Source: CAD feature listing. Evaluate the final solid. Frame: model axes, mm. A direction names the side the tool comes from. Round coordinates to 2 decimals unless told otherwise and drop trailing zeros. Write each loop counter-clockwise with the first axis right and the second up, starting at its lowest first coordinate (ties: lowest second). Pieces come first, ordered by that corner, then holes. Notation, with made-up numbers: M 36.5,-33.75 L 54.5,-33.75 A29 ccw 54.5,-9.75 Z; hole C 15.5,69 d10. An arc over 180 degrees is marked long. Answer in a Markdown table with one row per item. Add a question column.
Item 1: Cut plane A-A on y = -27. Return loops of the section in (x, z).
Item 2: Cut plane C-C on x = 4. Return loops of the section in (y, z).
Item 3: Mould query, pull axis Z, two halves, no side actions, for faces 4 (the face through (24, 20, 19)), 5 (the face through (25, 0, 37)), 6 (the face through (6.141, -0.224, 38.797)). Classes: released by +Z, released by -Z, zero draft, split by the parting line, or undercut.
Item 4: Cut plane B-B on x = 35. Give the number of separate pieces and of enclosed holes in the cut face, and give its area (3 significant figures).
Item 5: Material intervals for probe 1 along Y at (x, z) = (4, 9.25); probe 2 along Y at (x, z) = (21.5, 21.5); probe 3 along Z at (x, y) = (7, -21), sorted ascending.
Item 6: Cut plane D-D on y = 10. Return loops of the section in (x, z).
Item 7: Set-up query: faces 1 (the face through (31, 5, 41)), 2 (the face through (39, -5, 41)), 3 (the face through (8, -27, 9)). Return all of +Z, -Z, +X, -X, +Y, -Y with unobstructed straight access to the full face (end or side cutting, diameter ignored); none if empty.
Item 8: Contact query for flat-ended pins moving along their axis: pin 1 (5 mm diameter, centred on x = 7, y = 1, fed in from +Z); pin 2 (1.5 mm diameter, centred on y = 18, z = 19, fed in from -X); pin 3 (2 mm diameter, centred on y = 3.5, z = 41.5, fed in from -X). Output: stop coordinate, or through.
from build123d import *

# Parameters (mm, degrees)
ESTRUSIONE_ESTRUSIONE1_DEPTH  = 10
SCHIZZO6_W                    = 8
SCHIZZO6_H                    = 8
SCHIZZO6_H_2                  = 2
ESTRUSIONE_ESTRUSIONE4_DEPTH  = 10
TAGLIO_ESTRUSIONE1_DEPTH      = 54.150729064
SCHIZZO4_W                    = 3
SCHIZZO4_H                    = 6
ESTRUSIONE_ESTRUSIONE2_DEPTH  = 3
SCHIZZO5_W                    = 3
SCHIZZO5_H                    = 6
ESTRUSIONE_ESTRUSIONE3_DEPTH  = 3
SCHIZZO3_W                    = 5
SCHIZZO3_H                    = 6
TAGLIO_ESTRUSIONE2_DEPTH      = 67.820655489
FORO_FILETTATO_M3X0_5_1_D     = 2.5
ESTRUSIONE_ESTRUSIONE5_DEPTH  = 30
SCHIZZO10_W                   = 3
SCHIZZO10_H                   = 34
ESTRUSIONE_ESTRUSIONE6_DEPTH  = 34
SCHIZZO18_W                   = 8
SCHIZZO18_H                   = 8
TAGLIO_ESTRUSIONE3_DEPTH      = 5
SCHIZZO24_W                   = 8
SCHIZZO24_H                   = 2
ESTRUSIONE_ESTRUSIONE9_DEPTH  = 5
SCHIZZO23_W                   = 8
SCHIZZO23_H                   = 8
TAGLIO_ESTRUSIONE4_DEPTH      = 5
SCHIZZO25_W                   = 8
SCHIZZO25_H                   = 2
ESTRUSIONE_ESTRUSIONE10_DEPTH = 5
FORO_FILETTATO_M3X0_5_4_D     = 2.5
FORO_FILETTATO_M3X0_5_4_DEPTH = 7.5
FORO_FILETTATO_M3X0_5_4_TIP   = 0.751075774
FORO_FILETTATO_M3X0_5_5_D     = 2.5
FORO_FILETTATO_M3X0_5_5_DEPTH = 7.5
FORO_FILETTATO_M3X0_5_5_TIP   = 0.751075774
SCHIZZO11_W                   = 2
SCHIZZO11_H                   = 15
ESTRUSIONE_ESTRUSIONE7_DEPTH  = 3
SCHIZZO12_W                   = 2
SCHIZZO12_H                   = 5
ESTRUSIONE_ESTRUSIONE8_DEPTH  = 3
SCHIZZO28_W                   = 8
SCHIZZO28_H                   = 2
ESTRUSIONE_ESTRUSIONE11_DEPTH = 2
SCHIZZO29_W                   = 8
SCHIZZO29_H                   = 2
ESTRUSIONE_ESTRUSIONE12_DEPTH = 2
RACCORDO1_R                   = 4
RACCORDO2_DEPTH               = 2
RACCORDO2_START               = 8
RACCORDO2_2_DEPTH             = 2
RACCORDO2_START_2             = -1
RACCORDO2_3_DEPTH             = 12
RACCORDO2_START_3             = -23
RACCORDO2_4_DEPTH             = 3
RACCORDO2_START_4             = 20
RACCORDO2_5_DEPTH             = 3
RACCORDO2_START_5             = 31
RACCORDO2_6_DEPTH             = 8
RACCORDO30_R                  = 2
SCHIZZO30_R                   = 7
TAGLIO_ESTRUSIONE5_DEPTH      = 17


with BuildPart() as part:
    # Schizzo1 → Estrusione-Estrusione1 (new body)
    with BuildSketch(Plane.XY):
        Polygon((0, -23), (42, -23), (42, -17), (8, -17), (8, 17), (42, 17), (42, 23), (0, 23), align=None)
    extrude(amount=ESTRUSIONE_ESTRUSIONE1_DEPTH)

    # Schizzo6 → Estrusione-Estrusione4 (add)
    with BuildSketch(Plane.XY.offset(10)):
        with Locations((4, -27)):
            Rectangle(SCHIZZO6_W, SCHIZZO6_H)
        with Locations((4, 27)):
            Rectangle(SCHIZZO6_W, SCHIZZO6_H)
        with Locations((35, -24)):
            Rectangle(SCHIZZO6_W, SCHIZZO6_H_2)
        with Locations((35, 24)):
            Rectangle(SCHIZZO6_W, SCHIZZO6_H_2)
    extrude(amount=-ESTRUSIONE_ESTRUSIONE4_DEPTH)

    # Schizzo2 → Taglio-Estrusione1 (cut, through all)
    with BuildSketch(Plane(origin=(42, 0, 0), x_dir=(0, 0, -1), z_dir=(1, 0, 0))):
        Polygon((-8, -23), (-8, -41.817102562), (-2, -41.817102562), (-2, -22.5), (-2, -20), (-8, -20), align=None)
    taglio_estrusione1 = extrude(amount=-TAGLIO_ESTRUSIONE1_DEPTH, mode=Mode.SUBTRACT)

    # Schizzo4 → Estrusione-Estrusione2 (add)
    with BuildSketch(Plane(origin=(0, -20, 0), x_dir=(-1, 0, 0), z_dir=(0, -1, 0))):
        with Locations((-40.5, -5)):
            Rectangle(SCHIZZO4_W, SCHIZZO4_H)
    extrude(amount=ESTRUSIONE_ESTRUSIONE2_DEPTH)

    # Specchia1: Taglio-Estrusione1 across plane
    add(taglio_estrusione1.mirror(Plane.ZX), mode=Mode.SUBTRACT)

    # Schizzo5 → Estrusione-Estrusione3 (add)
    with BuildSketch(Plane(origin=(0, 20, 0), x_dir=(1, 0, 0), z_dir=(0, 1, 0))):
        with Locations((40.5, -5)):
            Rectangle(SCHIZZO5_W, SCHIZZO5_H)
    extrude(amount=ESTRUSIONE_ESTRUSIONE3_DEPTH)

    # Schizzo3 → Taglio-Estrusione2 (cut, through all)
    with BuildSketch(Plane.XZ.offset(20)):
        with Locations((2.5, 5)):
            Rectangle(SCHIZZO3_W, SCHIZZO3_H)
    extrude(amount=-TAGLIO_ESTRUSIONE2_DEPTH, mode=Mode.SUBTRACT)

    # Foro filettato M3x0.5-1 (through all)
    with Locations(Plane.XY.offset(10)):
        with Locations((4, -27), (4, 27)):
            Hole(FORO_FILETTATO_M3X0_5_1_D / 2)

    # Schizzo9 → Estrusione-Estrusione5 (add)
    with BuildSketch(Plane.XY.offset(10)):
        Polygon((5, -20), (42, -20), (42, -17), (8, -17), (8, 17), (42, 17), (42, 20), (5, 20), align=None)
    extrude(amount=ESTRUSIONE_ESTRUSIONE5_DEPTH)

    # Schizzo10 → Estrusione-Estrusione6 (add)
    with BuildSketch(Plane(origin=(8, 0, 0), x_dir=(0, 0, -1), z_dir=(1, 0, 0))):
        with Locations((-38.5, 0)):
            Rectangle(SCHIZZO10_W, SCHIZZO10_H)
    extrude(amount=ESTRUSIONE_ESTRUSIONE6_DEPTH)

    # Schizzo18 → Taglio-Estrusione3 (cut)
    with BuildSketch(Plane.XZ.offset(25)):
        with Locations((35, 12)):
            Rectangle(SCHIZZO18_W, SCHIZZO18_H)
    extrude(amount=-TAGLIO_ESTRUSIONE3_DEPTH, mode=Mode.SUBTRACT)

    # Schizzo24 → Estrusione-Estrusione9 (add)
    with BuildSketch(Plane.XZ.offset(20)):
        with Locations((35, 15)):
            Rectangle(SCHIZZO24_W, SCHIZZO24_H)
    extrude(amount=ESTRUSIONE_ESTRUSIONE9_DEPTH)

    # Schizzo23 → Taglio-Estrusione4 (cut)
    with BuildSketch(Plane(origin=(0, 25, 0), x_dir=(1, 0, 0), z_dir=(0, 1, 0))):
        with Locations((35, -12)):
            Rectangle(SCHIZZO23_W, SCHIZZO23_H)
    extrude(amount=-TAGLIO_ESTRUSIONE4_DEPTH, mode=Mode.SUBTRACT)

    # Schizzo25 → Estrusione-Estrusione10 (add)
    with BuildSketch(Plane(origin=(0, 20, 0), x_dir=(1, 0, 0), z_dir=(0, 1, 0))):
        with Locations((35, -15)):
            Rectangle(SCHIZZO25_W, SCHIZZO25_H)
    extrude(amount=ESTRUSIONE_ESTRUSIONE10_DEPTH)

    # Foro filettato M3x0.5-4
    with Locations(Plane(origin=(0, -20, 0), x_dir=(-1, 0, 0), z_dir=(0, -1, 0))):
        with Locations((-35, -10)):
            Hole(FORO_FILETTATO_M3X0_5_4_D / 2, depth=FORO_FILETTATO_M3X0_5_4_DEPTH)
            with Locations((0, 0, -(FORO_FILETTATO_M3X0_5_4_DEPTH + FORO_FILETTATO_M3X0_5_4_TIP / 2))):  # 118° drill point
                Cone(0, FORO_FILETTATO_M3X0_5_4_D / 2, FORO_FILETTATO_M3X0_5_4_TIP, mode=Mode.SUBTRACT)

    # Foro filettato M3x0.5-5
    with Locations(Plane(origin=(0, 20, 0), x_dir=(1, 0, 0), z_dir=(0, 1, 0))):
        with Locations((35, -10)):
            Hole(FORO_FILETTATO_M3X0_5_5_D / 2, depth=FORO_FILETTATO_M3X0_5_5_DEPTH)
            with Locations((0, 0, -(FORO_FILETTATO_M3X0_5_5_DEPTH + FORO_FILETTATO_M3X0_5_5_TIP / 2))):  # 118° drill point
                Cone(0, FORO_FILETTATO_M3X0_5_5_D / 2, FORO_FILETTATO_M3X0_5_5_TIP, mode=Mode.SUBTRACT)

    # Schizzo11 → Estrusione-Estrusione7 (add)
    with BuildSketch(Plane.XY.offset(40)):
        with Locations((38, 0)):
            Rectangle(SCHIZZO11_W, SCHIZZO11_H)
        with Locations((32, 0)):
            Rectangle(SCHIZZO11_W, SCHIZZO11_H)
    extrude(amount=ESTRUSIONE_ESTRUSIONE7_DEPTH)

    # Schizzo12 → Estrusione-Estrusione8 (add)
    with BuildSketch(Plane.XY.offset(16)):
        with Locations((38, -22.5)):
            Rectangle(SCHIZZO12_W, SCHIZZO12_H)
        with Locations((32, -22.5)):
            Rectangle(SCHIZZO12_W, SCHIZZO12_H)
    estrusione_estrusione8 = extrude(amount=ESTRUSIONE_ESTRUSIONE8_DEPTH)

    # Schizzo28 → Estrusione-Estrusione11 (add)
    with BuildSketch(Plane.XZ.offset(23)):
        with Locations((27, 9)):
            Rectangle(SCHIZZO28_W, SCHIZZO28_H)
    extrude(amount=ESTRUSIONE_ESTRUSIONE11_DEPTH)

    # Schizzo29 → Estrusione-Estrusione12 (add)
    with BuildSketch(Plane(origin=(0, 23, 0), x_dir=(1, 0, 0), z_dir=(0, 1, 0))):
        with Locations((27, -9)):
            Rectangle(SCHIZZO29_W, SCHIZZO29_H)
    extrude(amount=ESTRUSIONE_ESTRUSIONE12_DEPTH)

    # Specchia2: Estrusione-Estrusione8 across plane
    add(estrusione_estrusione8.mirror(Plane.ZX))

    # Raccordo1
    raccordo1_edges = [part.edges().sort_by_distance(p)[0] for p in [
        (23.5, -20, 40),
        (23.5, 20, 40),
        (5, 0, 40),
        (5, 20, 25),
        (5, -20, 25),
        (42, 20, 0),
        (42, -20, 0),
        (25, -17, 37),
        (25, -17, 0),
        (25, 17, 37),
        (25, 17, 0),
    ]]
    fillet(raccordo1_edges, radius=RACCORDO1_R)

    # Raccordo2: read off the stored shape, not the designer's step
    # Raccordo2 outline → Raccordo2 (add)
    with BuildSketch(Plane.XY):
        with BuildLine():
            Line((8, -23), (8, -26))
            ThreePointArc((8, -26), (8.878679656, -23.878679656), (11, -23))
            Line((11, -23), (8, -23))
        make_face()
        with BuildLine():
            Line((8, 23), (11, 23))
            ThreePointArc((11, 23), (8.878679656, 23.878679656), (8, 26))
            Line((8, 26), (8, 23))
        make_face()
        with BuildLine():
            Line((31, 23), (31, 25))
            ThreePointArc((31, 25), (29.903623683, 23.550510257), (28.171572875, 23))
            Line((28.171572875, 23), (31, 23))
        make_face()
        with BuildLine():
            ThreePointArc((28.171572875, -23), (29.903623683, -23.550510257), (31, -25))
            Line((31, -25), (31, -23))
            Line((31, -23), (28.171572875, -23))
        make_face()
    extrude(amount=RACCORDO2_DEPTH)

    # Raccordo2 2 outline → Raccordo2 2 (add)
    with BuildSketch(Plane.XY.offset(RACCORDO2_START)):
        with BuildLine():
            ThreePointArc((23, 25), (21.903623683, 23.550510257), (20.171572875, 23))
            Line((20.171572875, 23), (23, 23))
            Line((23, 23), (23, 25))
        make_face()
        with BuildLine():
            Line((23, -23), (20.171572875, -23))
            ThreePointArc((20.171572875, -23), (21.903623683, -23.550510257), (23, -25))
            Line((23, -25), (23, -23))
        make_face()
        with BuildLine():
            Line((8, -23), (8, -26))
            ThreePointArc((8, -26), (8.878679656, -23.878679656), (11, -23))
            Line((11, -23), (8, -23))
        make_face()
        with BuildLine():
            Line((8, 23), (11, 23))
            ThreePointArc((11, 23), (8.878679656, 23.878679656), (8, 26))
            Line((8, 26), (8, 23))
        make_face()
    extrude(amount=RACCORDO2_2_DEPTH)

    # Raccordo2 3 outline → Raccordo2 3 (cut)
    with BuildSketch(Plane.XY.offset(RACCORDO2_START_2)):
        with BuildLine():
            ThreePointArc((8, -28), (7.121320344, -30.121320344), (5, -31))
            Line((5, -31), (8, -31))
            Line((8, -31), (8, -28))
        make_face()
        with BuildLine():
            ThreePointArc((3, -31), (0.878679656, -30.121320344), (0, -28))
            Line((0, -28), (0, -31))
            Line((0, -31), (3, -31))
        make_face()
        with BuildLine():
            ThreePointArc((0, 28), (0.878679656, 30.121320344), (3, 31))
            Line((3, 31), (0, 31))
            Line((0, 31), (0, 28))
        make_face()
        with BuildLine():
            ThreePointArc((5, 31), (7.121320344, 30.121320344), (8, 28))
            Line((8, 28), (8, 31))
            Line((8, 31), (5, 31))
        make_face()
    extrude(amount=RACCORDO2_3_DEPTH, mode=Mode.SUBTRACT)

    # Raccordo2 4 outline → Raccordo2 4 (cut)
    with BuildSketch(Plane(origin=(0, 0, 0), x_dir=(1, 0, 0), z_dir=(0, 1, 0)).offset(RACCORDO2_START_3)):
        with BuildLine():
            ThreePointArc((42, -7), (41.121320344, -9.121320344), (39, -10))
            Line((39, -10), (42, -10))
            Line((42, -10), (42, -7))
        make_face()
    extrude(amount=RACCORDO2_4_DEPTH, mode=Mode.SUBTRACT)

    # Raccordo2 5 outline → Raccordo2 5 (cut)
    with BuildSketch(Plane(origin=(0, 0, 0), x_dir=(1, 0, 0), z_dir=(0, 1, 0)).offset(RACCORDO2_START_4)):
        with BuildLine():
            ThreePointArc((42, -7), (41.121320344, -9.121320344), (39, -10))
            Line((39, -10), (42, -10))
            Line((42, -10), (42, -7))
        make_face()
    extrude(amount=RACCORDO2_5_DEPTH, mode=Mode.SUBTRACT)

    # Raccordo2 6 outline → Raccordo2 6 (cut)
    with BuildSketch(Plane.YZ.offset(RACCORDO2_START_5)):
        with BuildLine():
            ThreePointArc((22, 19), (24.121320344, 18.121320344), (25, 16))
            Line((25, 16), (25, 19))
            Line((25, 19), (22, 19))
        make_face()
        with BuildLine():
            ThreePointArc((-7.5, 40), (-6.621320344, 42.121320344), (-4.5, 43))
            Line((-4.5, 43), (-7.5, 43))
            Line((-7.5, 43), (-7.5, 40))
        make_face()
        with BuildLine():
            ThreePointArc((4.5, 43), (6.621320344, 42.121320344), (7.5, 40))
            Line((7.5, 40), (7.5, 43))
            Line((7.5, 43), (4.5, 43))
        make_face()
        with BuildLine():
            Line((-25, 19), (-25, 16))
            ThreePointArc((-25, 16), (-24.121320344, 18.121320344), (-22, 19))
            Line((-22, 19), (-25, 19))
        make_face()
    extrude(amount=RACCORDO2_6_DEPTH, mode=Mode.SUBTRACT)

    # Raccordo30
    raccordo30_edges = [part.edges().sort_by_distance(p)[0] for p in [
        (39, 23, 1.063508327),
        (39, -23, 1.063508327),
    ]]
    fillet(raccordo30_edges, radius=RACCORDO30_R - 0.0001)  # a hair under: the kernel refuses the full size

    # Schizzo30 → Taglio-Estrusione5 (cut)
    with BuildSketch(Plane(origin=(42, 0, 0), x_dir=(0, 0, -1), z_dir=(1, 0, 0))):
        with Locations((-47, 0)):
            Circle(SCHIZZO30_R)
    extrude(amount=-TAGLIO_ESTRUSIONE5_DEPTH, mode=Mode.SUBTRACT)


solid = part.part
Results below:
| question | item | result |
|---|---|---|
| 1 | outline | M 0,0 L 2.75,0 L 2.75,2 L 0,2 Z; M 0,8 L 2.75,8 L 2.75,10 L 0,10 Z; M 5.25,0 L 8,0 L 8,2 L 5.25,2 Z; M 5.25,8 L 8,8 L 8,10 L 5.25,10 Z |
| 2 | outline | M -31,0 L -28.25,0 L -28.25,2 L -31,2 Z; M -31,8 L -28.25,8 L -28.25,10 L -31,10 Z; M -25.75,0 L 25.75,0 L 25.75,2 L -25.75,2 Z; M -25.75,8 L 25.75,8 L 25.75,10 L -25.75,10 Z; M 28.25,0 L 31,0 L 31,2 L 28.25,2 Z; M 28.25,8 L 31,8 L 31,10 L 28.25,10 Z |
| 3 | face 4 | undercut |
| 3 | face 5 | released by -Z |
| 3 | face 6 | released by +Z |
| 4 | separate pieces | 3 |
| 4 | enclosed holes | 0 |
| 4 | area | 360 mm2 |
| 5 | probe 1 | -31 to -28.25, -25.75 to 25.75, 28.25 to 31 |
| 5 | probe 2 | -20 to -17, 17 to 20 |
| 5 | probe 3 | 0 to 2, 8 to 10 |
| 6 | outline | M 0,0 L 8,0 L 8,37 L 42,37 L 42,40 L 9,40 A4 ccw 5,36 L 5,10 L 0,10 L 0,8 L 5,8 L 5,2 L 0,2 Z |
| 7 | face 1 | +Z, -X, +Y, -Y |
| 7 | face 2 | +Z, +X, +Y, -Y |
| 7 | face 3 | +Z, -Z, +X, -Y |
| 8 | pin 1 | z = 40 |
| 8 | pin 2 | x = 5.2 |
| 8 | pin 3 | x = 31 |
